Read the model definition and answer for the solid it produces. Units are mm, in the model's axes. Coordinates: 2 decimals unless noted, no trailing zeros. Write each loop counter-clockwise with the first axis right and the second up, starting at its lowest first coordinate (ties: lowest second). Pieces come first, ordered by that corner, then holes.
1) The part is cut by section B-B (y = 206.5). Determine the outline of the cut face in (x, z).
2) Find the intervals of material crossed by line 1 (X direction, y = 182.5, z = -5.5), in increasing order.
3) The part is cut by section A-A (z = -3.75). Determine the outline of the cut face in (x, y), then the cut area to 3 significant figures.
4) Each of these flat-tipped pins is pushed along its axis until it touches: pin 1 Ø5.5 at (y, z) = (45, -1) entering from -X; pin 2 Ø9 at (x, z) = (635, -2.5) entering from +Y; pin 3 Ø9 at (x, z) = (-12.5, -2.5) entering from -Y. Where does it stop, or does it pass through?
from build123d import *

# Parameters (mm, degrees)
F1_DEPTH = 9.2075


with BuildPart() as f1:
    # F0 (on Top) → F1 (new body, symmetric)
    with BuildSketch(Plane.XY):
        Polygon((0, 136.8044), (0, 0), (621.284, 0), (621.284, 136.8044), (640.334, 136.8044), (640.334, 174.9044), (621.284, 174.9044), (621.284, 258.7244), (640.334, 258.7244), (640.334, 296.8244), (621.284, 296.8244), (621.284, 384.2766), (0, 384.2766), (0, 296.8244), (-19.05, 296.8244), (-19.05, 258.7244), (0, 258.7244), (0, 174.9044), (-19.05, 174.9044), (-19.05, 136.8044), align=None)
    extrude(amount=F1_DEPTH, both=True)


solid = f1.part
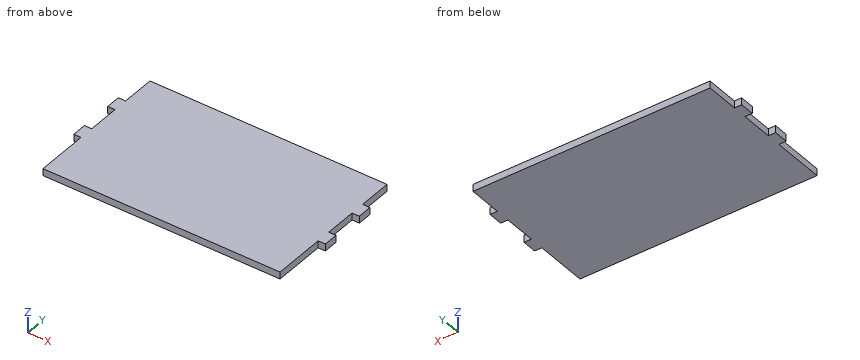
Reported:
1. outline: (0, -9.21) - (621.28, -9.21) - (621.28, 9.21) - (0, 9.21) - close
2. line 1: x = 0 to 621.28
3. outline: (-19.05, 136.8) - (0, 136.8) - (0, 0) - (621.28, 0) - (621.28, 136.8) - (640.33, 136.8) - (640.33, 174.9) - (621.28, 174.9) - (621.28, 258.72) - (640.33, 258.72) - (640.33, 296.82) - (621.28, 296.82) - (621.28, 384.28) - (0, 384.28) - (0, 296.82) - (-19.05, 296.82) - (-19.05, 258.72) - (0, 258.72) - (0, 174.9) - (-19.05, 174.9) - close
3. area: 242,000 mm2
4. pin 1: stops at x = 0
4. pin 2: stops at y = 296.82
4. pin 3: stops at y = 136.8
